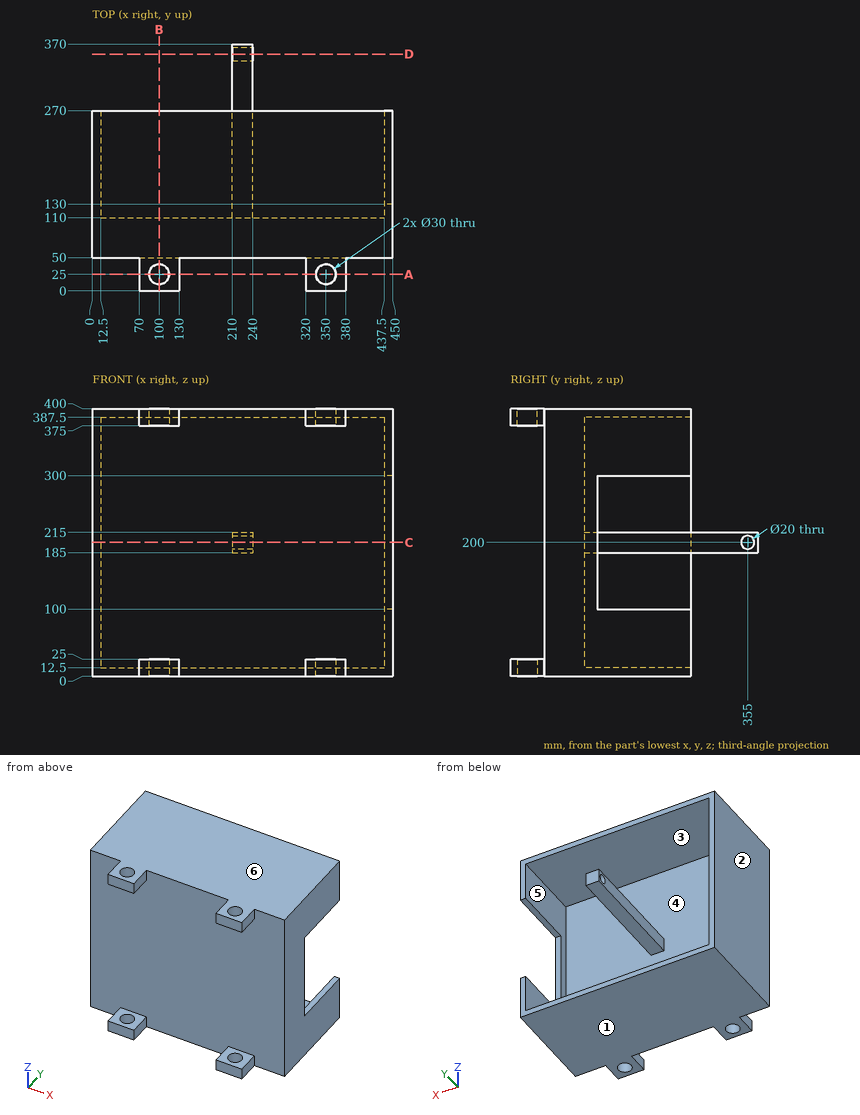
Geometry check sheet. Reference: drawing and pictorial views, mm from the part's lowest x, y, z. A direction names the side the tool comes from. Round coordinates to 2 decimals unless told otherwise and drop trailing zeros. Loops run counter-clockwise (first coordinate to the right, second up) from the corner with the lowest first, then second, coordinate; pieces in that order, holes last. Notation, with made-up numbers: (-4.5, 25) -> (48.5, 25) arc R7 cw to (48.5, 30) -> close; hole circle Ø4 at (58.25, -9). An arc over 180 degrees is marked (long way). Answer as a JSON object with one key per item and string values.
Q1. Go/stop test with flat-tipped pins: P1, Ø15, axis at x = 229, y = 291, coming from the +Z side; P2, Ø8, axis at y = 49.5, z = 109, coming from the +X side; P3, Ø20, axis at y = 17, z = 387, coming from the +X side; P4, Ø3, axis at x = 92, z = 356.5, coming from the -Y side. Record where each tip stops, or that it passes through.
Data:
{"P1": "stops at z = 215", "P2": "stops at x = 450", "P3": "stops at x = 380", "P4": "stops at y = 50"}
Q2. Section check D-D (y = 355). Record the boundary of the cut face in (x, z), then the cut area to 3 significant figures.
Data:
{"outline": "(210, 185) -> (240, 185) -> (240, 190) -> (210, 190) -> close; (210, 210) -> (240, 210) -> (240, 215) -> (210, 215) -> close", "area": "300 mm2"}
Q3. Section check A-A (y = 25). State how many separate pieces and enclosed holes the cut face has, then the cut area to 3 significant figures.
Data:
{"separate pieces": "8", "enclosed holes": "0", "area": "3,000 mm2"}
Q4. Draft check along Z on the marked faces 1, 2, 3 and 4. Enter one of: pulls with the +Z half, pulls with the -Z half, needs draft (parallel to the pull), parting line crosses it, or undercut.
Data:
{"face 1": "pulls with the -Z half", "face 2": "needs draft", "face 3": "undercut", "face 4": "undercut"}
Q5. Section check B-B (x = 100). Record the boundary of the cut face in (y, z), then the cut area to 3 significant figures.
Data:
{"outline": "(0, 0) -> (10, 0) -> (10, 25) -> (0, 25) -> close; (0, 375) -> (10, 375) -> (10, 400) -> (0, 400) -> close; (40, 0) -> (270, 0) -> (270, 12.5) -> (110, 12.5) -> (110, 387.5) -> (270, 387.5) -> (270, 400) -> (40, 400) -> (40, 375) -> (50, 375) -> (50, 25) -> (40, 25) -> close", "area": "29,000 mm2"}
Q6. Section check C-C (z = 200). Record the boundary of the cut face in (x, y).
Data:
{"outline": "(0, 50) -> (450, 50) -> (450, 130) -> (437.5, 130) -> (437.5, 110) -> (240, 110) -> (240, 345) -> (210, 345) -> (210, 110) -> (12.5, 110) -> (12.5, 270) -> (0, 270) -> close; (210, 365) -> (240, 365) -> (240, 370) -> (210, 370) -> close"}
Q7. Scan lines: line 1 (Z direction, x = 231, y = 257); line 2 (Y direction, x = 350, z = 394); line 3 (Z direction, x = 28.5, y = 111). Record each from-to range of solid material in increasing order. Write a range as from..to.
Data:
{"line 1": "z = 0..12.5, 185..215, 387.5..400", "line 2": "y = 0..10, 40..270", "line 3": "z = 0..12.5, 387.5..400"}
Q8. Access from +Z, -Z, +X, -X, +Y, -Y to the whole of each face (thin tool, end or side, straight path). Record for the marked faces 5 and 6.
Data:
{"face 5": "+Y", "face 6": "+Z, +X, -X, +Y, -Y"}
